Autodesk Inventor part; units mm, degrees
ref_plane "YZ Plane" through (0, 0, 0) normal (1, 0, 0) x (0, 1, 0)
ref_plane "XZ Plane" through (0, 0, 0) normal (0, 1, 0) x (-1, 0, 0)
ref_plane "XY Plane" through (0, 0, 0) normal (0, 0, 1) x (1, 0, 0)
sketch "스케치1" plane through (0, 0, 0) normal (0, 0, 1) x (1, 0, 0)
  line L0 (0, 0) -> (-35.14, 0)
  line L1 (-35.14, 0) -> (61.6, 0)
  line L2 (0, 35.14) -> (0, -35.14)
  line L3 (-35.14, -35.14) -> (61.6, -35.14)
  line L4 (61.6, -35.14) -> (61.6, 35.14)
  line L5 (61.6, 35.14) -> (-35.14, 35.14)
  line L6 (-35.14, 35.14) -> (-35.14, -35.14)
  line L7 (0, 0) -> (-27.87, 0)
  line L8 (0, 0) -> (42, 0)
  line L9 (42, 20) -> (42, -20)
  circle A0 centre (42, -20) radius 1.25
  circle A1 centre (42, 20) radius 1.25
  line L10 (0, 0) -> (45.5, 0)
  circle A2 centre (45.5, 0) radius 9
  circle A3 centre (45.5, 0) radius 16.1
  circle A4 centre (42, -20) radius 3
  circle A5 centre (42, 20) radius 3
  line L11 (45.5, 0) -> (61.6, 0) construction
  line L12 (42, 20) -> (45, 20) construction
  line L13 (44.1213, 22.1213) -> (55.8489, 12.3333)
  line L14 (42, 23) -> (0, 35.14)
  line L15 (-27.87, 28) -> (-27.87, -28)
  circle A6 centre (-27.87, 28) radius 1.25
  circle A7 centre (-27.87, 28) radius 3
  circle A8 centre (-27.87, -28) radius 1.25
  circle A9 centre (-27.87, -28) radius 3
  line L16 (-27.87, 31) -> (0, 35.14)
  line L17 (-30.87, 28) -> (-35.14, 0)
  line L18 (44.1213, -22.1213) -> (55.8489, -12.3333)
  line L19 (42, -23) -> (0, -35.14)
  line L20 (-27.87, -31) -> (0, -35.14)
  line L21 (-30.87, -28) -> (-35.14, 0)
  dimension "d20" = 6
  dimension "d0" = 35.14
  dimension "d1" = 96.74
  dimension "d3" = 70.28
  dimension "d4" = 27.87
  dimension "d9" = 42
  dimension "d11" = 40
  dimension "d12" = 2.5
  dimension "d13" = 2.5
  dimension "d14" = 45.5
  dimension "d15" = 18
  dimension "d16" = 32.2
  dimension "d19" = 6
  dimension "d27" = 56
  dimension "d28" = 2.5
  dimension "d29" = 6
  dimension "d30" = 2.5
  dimension "d31" = 6
extrude "돌출1" add sketch "스케치1" along normal blind 5.5 contours L2 L20 A9 L15 L0 | L2 L14 A5 L9 A3 L1 | L0 L15 A7 L16 L2 | L1 A3 L9 A4 L19 L2 | L15 A9 L21 L0 | L0 L17 A7 L15 | A3 L9 A2 L1 | L1 A2 L9 A3 | A3 L1 A2 L9 | L18 A4 L9 A3 | A7 | A9 | A2 L9 L1 | L1 L9 A2 | L9 A5 L13 A3 | L9 A2 L1 A3 | A5 | A4 | L9 A2 L1 | L1 A2 L9
sketch "스케치2" plane through (0, 0, 5.5) normal (0, 0, 1) x (1, 0, 0)
  line L0 (0, 0) -> (-35.14, 0)
  line L1 (-35.14, 0) -> (61.6, 0)
  line L2 (0, 35.14) -> (0, -35.14)
  line L3 (-35.14, -35.14) -> (61.6, -35.14)
  line L4 (61.6, -35.14) -> (61.6, 35.14)
  line L5 (61.6, 35.14) -> (-35.14, 35.14)
  line L6 (-35.14, 35.14) -> (-35.14, -35.14)
  line L7 (0, 0) -> (-27.87, 0)
  line L8 (0, 0) -> (42, 0)
  line L9 (42, 20) -> (42, -20)
  circle A0 centre (42, -20) radius 1.25
  circle A1 centre (42, 20) radius 1.25
  line L10 (0, 0) -> (45.5, 0)
  circle A2 centre (45.5, 0) radius 9
  circle A3 centre (45.5, 0) radius 16.1
  circle A4 centre (42, -20) radius 3
  circle A5 centre (42, 20) radius 3
  line L11 (45.5, 0) -> (61.6, 0) construction
  line L12 (42, 20) -> (45, 20) construction
  line L13 (44.1213, 22.1213) -> (55.8489, 12.3333)
  line L14 (42, 23) -> (0, 35.14)
  line L15 (-27.87, 28) -> (-27.87, -28)
  circle A6 centre (-27.87, 28) radius 1.25
  circle A7 centre (-27.87, 28) radius 3
  circle A8 centre (-27.87, -28) radius 1.25
  circle A9 centre (-27.87, -28) radius 3
  line L16 (-27.87, 31) -> (0, 35.14)
  line L17 (-30.87, 28) -> (-35.14, 0)
  line L18 (-27.87, -31) -> (0, -35.14)
  line L19 (-30.87, -28) -> (-35.14, 0)
  line L20 (42, -23) -> (0, -35.14)
  line L21 (44.1213, -22.1213) -> (55.8489, -12.3333)
  point P0 (55.7837, -12.3877)
  point P1 (55.7837, 12.3877)
  dimension "d46" = 6
  dimension "d34" = 35.14
  dimension "d35" = 96.74
  dimension "d36" = 70.28
  dimension "d37" = 27.87
  dimension "d38" = 42
  dimension "d39" = 40
  dimension "d40" = 2.5
  dimension "d41" = 2.5
  dimension "d42" = 45.5
  dimension "d43" = 18
  dimension "d44" = 32.2
  dimension "d45" = 6
  dimension "d47" = 56
  dimension "d48" = 2.5
  dimension "d49" = 6
  dimension "d50" = 2.5
  dimension "d51" = 6
extrude "돌출2" add sketch "스케치2" along normal blind 15 contours A3 L9 A2 L1 | L1 A2 L9 A3 | A3 L1 A2 L9 | A7 | A9 | A2 L9 L1 | L1 L9 A2 | L9 A2 L1 A3 | A5 | A4 | L9 A2 L1 | L1 A2 L9
sketch "스케치3" plane through (0, 0, 20.5) normal (0, 0, 1) x (1, 0, 0)
  line L0 (0, 0) -> (-35.14, 0)
  line L1 (-35.14, 0) -> (61.6, 0)
  line L2 (0, 35.14) -> (0, -35.14)
  line L3 (-35.14, -35.14) -> (61.6, -35.14)
  line L4 (61.6, -35.14) -> (61.6, 35.14)
  line L5 (61.6, 35.14) -> (-35.14, 35.14)
  line L6 (-35.14, 35.14) -> (-35.14, -35.14)
  line L7 (0, 0) -> (-27.87, 0)
  line L8 (0, 0) -> (42, 0)
  line L9 (42, 20) -> (42, -20)
  circle A0 centre (42, -20) radius 1.25
  circle A1 centre (42, 20) radius 1.25
  line L10 (0, 0) -> (45.5, 0)
  circle A2 centre (45.5, 0) radius 9
  circle A3 centre (45.5, 0) radius 16.1
  circle A4 centre (42, -20) radius 3
  circle A5 centre (42, 20) radius 3
  line L11 (45.5, 0) -> (61.6, 0) construction
  line L12 (42, 20) -> (45, 20) construction
  line L13 (44.1213, 22.1213) -> (55.8489, 12.3333)
  line L14 (42, 23) -> (0, 35.14)
  line L15 (-27.87, 28) -> (-27.87, -28)
  circle A6 centre (-27.87, 28) radius 1.25
  circle A7 centre (-27.87, 28) radius 3
  circle A8 centre (-27.87, -28) radius 1.25
  circle A9 centre (-27.87, -28) radius 3
  line L16 (-27.87, 31) -> (0, 35.14)
  line L17 (-30.87, 28) -> (-35.14, 0)
  line L18 (-27.87, -31) -> (0, -35.14)
  line L19 (-30.87, -28) -> (-35.14, 0)
  line L20 (42, -23) -> (0, -35.14)
  line L21 (44.1213, -22.1213) -> (55.8489, -12.3333)
  point P0 (42, -15.715)
  point P1 (55.7837, -12.3877)
  point P2 (55.7837, 12.3877)
  point P3 (42, 15.715)
  point P4 (42, 17)
  point P5 (42, -17)
  dimension "d66" = 6
  dimension "d54" = 35.14
  dimension "d55" = 96.74
  dimension "d56" = 70.28
  dimension "d57" = 27.87
  dimension "d58" = 42
  dimension "d59" = 40
  dimension "d60" = 2.5
  dimension "d61" = 2.5
  dimension "d62" = 45.5
  dimension "d63" = 18
  dimension "d64" = 32.2
  dimension "d65" = 6
  dimension "d67" = 56
  dimension "d68" = 2.5
  dimension "d69" = 6
  dimension "d70" = 2.5
  dimension "d71" = 6
extrude "돌출3" add sketch "스케치3" along normal blind 1.6 contours L2 L18 A9 L15 L0 | L2 L14 A5 L9 A3 L1 | L0 L15 A7 L16 L2 | L1 A3 L9 A4 L20 L2 | L15 A9 L19 L0 | L0 L17 A7 L15 | A3 L9 A2 L1 | L1 A2 L9 A3 | A3 L1 A2 L9 | A7 | A9 | A2 L9 L1 | L1 L9 A2 | L9 A2 L1 A3 | A5 | A4 | L9 A2 L1 | L1 A2 L9
sketch "스케치4" plane through (0, 0, 22.1) normal (0, 0, 1) x (1, 0, 0)
  line L0 (0, 0) -> (-35.14, 0)
  line L1 (-35.14, 0) -> (61.6, 0)
  line L2 (0, 35.14) -> (0, -35.14)
  line L3 (-35.14, -35.14) -> (61.6, -35.14)
  line L4 (61.6, -35.14) -> (61.6, 35.14)
  line L5 (61.6, 35.14) -> (-35.14, 35.14)
  line L6 (-35.14, 35.14) -> (-35.14, -35.14)
  line L7 (0, 0) -> (-27.87, 0)
  line L8 (0, 0) -> (42, 0)
  line L9 (42, 20) -> (42, -20)
  circle A0 centre (42, -20) radius 1.25
  circle A1 centre (42, 20) radius 1.25
  line L10 (0, 0) -> (45.5, 0)
  circle A2 centre (45.5, 0) radius 9
  circle A3 centre (45.5, 0) radius 16.1
  circle A4 centre (42, -20) radius 3
  circle A5 centre (42, 20) radius 3
  line L11 (45.5, 0) -> (61.6, 0) construction
  line L12 (42, 20) -> (45, 20) construction
  line L13 (44.1213, 22.1213) -> (55.8489, 12.3333)
  line L14 (42, 23) -> (0, 35.14)
  line L15 (-27.87, 28) -> (-27.87, -28)
  circle A6 centre (-27.87, 28) radius 1.25
  circle A7 centre (-27.87, 28) radius 3
  circle A8 centre (-27.87, -28) radius 1.25
  circle A9 centre (-27.87, -28) radius 3
  line L16 (-27.87, 31) -> (0, 35.14)
  line L17 (-30.87, 28) -> (-35.14, 0)
  line L18 (-27.87, -31) -> (0, -35.14)
  line L19 (-30.87, -28) -> (-35.14, 0)
  line L20 (42, -23) -> (0, -35.14)
  line L21 (44.1213, -22.1213) -> (55.8489, -12.3333)
  dimension "d86" = 6
  dimension "d74" = 35.14
  dimension "d75" = 96.74
  dimension "d76" = 70.28
  dimension "d77" = 27.87
  dimension "d78" = 42
  dimension "d79" = 40
  dimension "d80" = 2.5
  dimension "d81" = 2.5
  dimension "d82" = 45.5
  dimension "d83" = 18
  dimension "d84" = 32.2
  dimension "d85" = 6
  dimension "d87" = 56
  dimension "d88" = 2.5
  dimension "d89" = 6
  dimension "d90" = 2.5
  dimension "d91" = 6
extrude "돌출4" add sketch "스케치4" along normal blind 10 contours A7 | A9 | A5 | A4
sketch "스케치5" plane through (0, 0, 0) normal (0, 0, -1) x (-1, 0, 0)
  line L0 (27.87, -31) -> (0, -35.14)
  arc A0 (27.87, -31) -> (30.87, -28) centre (27.87, -28) ccw
  line L1 (35.14, 0) -> (30.87, -28)
  line L2 (30.87, 28) -> (35.14, 0)
  arc A1 (30.87, 28) -> (27.87, 31) centre (27.87, 28) ccw
  line L3 (0, 35.14) -> (27.87, 31)
  line L4 (-42, 23) -> (0, 35.14)
  arc A2 (-42, 23) -> (-44.1213, 22.1213) centre (-42, 20) ccw
  line L5 (-55.8489, 12.3333) -> (-44.1213, 22.1213)
  arc A3 (-55.8489, 12.3333) -> (-55.8489, -12.3333) centre (-45.5, 0) ccw
  line L6 (-44.1213, -22.1213) -> (-55.8489, -12.3333)
  arc A4 (-44.1213, -22.1213) -> (-42, -23) centre (-42, -20) ccw
  line L7 (0, -35.14) -> (-42, -23)
  circle A5 centre (-42, 20) radius 1.25
  circle A6 centre (27.87, 28) radius 1.25
  circle A7 centre (27.87, -28) radius 1.25
  circle A8 centre (-42, -20) radius 1.25
  line L8 (0, -35.14) -> (0, 35.14)
  line L9 (0, 0) -> (-45.5, 0)
  circle A9 centre (0, 0) radius 2.5
  circle A10 centre (-45.5, 0) radius 2.5
  dimension "d94" = 5
  dimension "d95" = 5
extrude "돌출5" add sketch "스케치5" along normal blind 2 contours A10 | A9 L9 L8 | L8 A9 | L9 A9 L8
sketch "스케치6" plane through (0, 0, 22.1) normal (0, 0, 1) x (1, 0, 0)
  arc A0 (42, -17) -> (42, -23) centre (42, -20) ccw
  line L0 (42, -17) -> (42, -15.715)
  arc A1 (42, -15.715) -> (55.7837, -12.3877) centre (45.5, 0) ccw
  line L1 (55.7837, -12.3877) -> (55.8489, -12.3333)
  arc A2 (55.8489, -12.3333) -> (55.8489, 12.3333) centre (45.5, 0) ccw
  line L2 (55.8489, 12.3333) -> (55.7837, 12.3877)
  arc A3 (55.7837, 12.3877) -> (42, 15.715) centre (45.5, 0) ccw
  line L3 (42, 15.715) -> (42, 17)
  arc A4 (42, 23) -> (42, 17) centre (42, 20) ccw
  line L4 (42, 23) -> (0, 35.14)
  line L5 (0, 35.14) -> (-27.87, 31)
  arc A5 (-30.87, 28) -> (-27.87, 31) centre (-27.87, 28) ccw
  line L6 (-30.87, 28) -> (-35.14, 0)
  line L7 (-35.14, 0) -> (-30.87, -28)
  arc A6 (-27.87, -31) -> (-30.87, -28) centre (-27.87, -28) ccw
  line L8 (-27.87, -31) -> (0, -35.14)
  line L9 (0, -35.14) -> (42, -23)
  circle A7 centre (-27.87, 28) radius 3
  circle A8 centre (-27.87, 28) radius 1.25
  circle A9 centre (-27.87, -28) radius 3
  circle A10 centre (-27.87, -28) radius 1.25
  circle A11 centre (42, -20) radius 1.25
  circle A12 centre (42, -20) radius 3
  circle A13 centre (42, -20) radius 1.25
  circle A14 centre (42, 20) radius 3
  circle A15 centre (42, 20) radius 1.25
  line L10 (-27.87, 28) -> (-27.87, 24.6)
  line L11 (-27.87, 24.6) -> (-9.87, 24.6)
  line L12 (-9.87, 24.6) -> (10.13, 24.6)
  line L13 (10.13, 24.6) -> (10.13, 29.6)
  line L14 (10.13, 29.6) -> (-9.87, 29.6)
  line L15 (-9.87, 29.6) -> (-9.87, 24.6)
  line L16 (-9.87, 29.6) -> (-7.87, 29.6)
  line L17 (-7.87, 29.6) -> (-9.87, 27.6)
  line L18 (10.13, 29.6) -> (8.13, 29.6)
  line L19 (8.13, 29.6) -> (10.13, 27.6)
  point P0 (0, 0)
  dimension "d98" = 3.4
  dimension "d99" = 18
  dimension "d100" = 20
  dimension "d101" = 5
  dimension "d102" = 2
  dimension "d103" = 45
  dimension "d104" = 2
extrude "돌출6" add sketch "스케치6" along normal blind 5 contours L15 L17 L14 L19 L13 L12
sketch "스케치7" plane through (0, 0, 27.1) normal (0, 0, 1) x (1, 0, 0)
  line L0 (8.13, 29.6) -> (-7.87, 29.6)
  line L1 (-7.87, 29.6) -> (-9.87, 27.6)
  line L2 (-9.87, 27.6) -> (-9.87, 24.6)
  line L3 (-9.87, 24.6) -> (10.13, 24.6)
  line L4 (10.13, 24.6) -> (10.13, 27.6)
  line L5 (10.13, 27.6) -> (8.13, 29.6)
  line L6 (-9.37, 27.3929) -> (-7.6629, 29.1)
  line L7 (-7.6629, 29.1) -> (7.9229, 29.1)
  line L8 (7.9229, 29.1) -> (9.63, 27.3929)
  line L9 (9.63, 27.3929) -> (9.63, 25.1)
  line L10 (9.63, 25.1) -> (-9.37, 25.1)
  line L11 (-9.37, 25.1) -> (-9.37, 27.3929)
  point P0 (0, 0)
  dimension "d107" = 0.5
extrude "돌출7" cut sketch "스케치7" against normal blind 5 contours L6 L7 L8 L9 L10 L11
properties part number "base"
Geometry check sheet. Reference: the model listing, model coordinates, mm. A direction names the side the tool comes from. Give positions to 0.01 mm unless a question says otherwise; leave off trailing zeros. Write each loop counter-clockwise with the first axis right and the second up, starting at its lowest first coordinate (ties: lowest second). Pieces come first, ordered by that corner, then holes. Notation, with made-up numbers: (51, -20.5) - (106, -20.5) arc R25 cw to (106, 1.5) - close; hole circle Ø6 at (-39.75, 20.5). An arc over 180 degrees is marked (long way). Put each result on its own line as item: value.
1. Draft check along X on faces 1 (the flat face through (-8.86, 28.61, 24.56)), 2 (the flat face through (46, 0, -2)), 3 (the flat face through (-14.13, -33.04, 2.71)), 4 (the flat face through (10.13, 26, 25)). Enter one of: +X half, -X half, draft (parallel to the pull), parting line (faces both ways), or undercut.
Ans:
face 1: undercut
face 2: draft
face 3: -X half
face 4: +X half
2. Sectioned sample at A-A, the plane z = 10. Give the number of separate pieces and of enclosed holes in the cut face, plus the area to 3 significant figures.
Ans:
separate pieces: 5
enclosed holes: 4
area: 908 mm²
3. Sectioned sample at B-B, the plane x = -15. Enter the section's corners in (y, z), plus the area to 3 significant figures.
Ans:
outline: (-32.91, 0) - (32.91, 0) - (32.91, 5.5) - (-32.91, 5.5) - close; (-32.91, 20.5) - (32.91, 20.5) - (32.91, 22.1) - (-32.91, 22.1) - close
area: 467 mm²
4. Sectioned sample at D-D, the plane z = 4. Enter the section's corners in (x, y), plus the area to 3 significant figures.
Ans:
outline: (-35.14, 0) - (-30.87, -28) arc R3 ccw to (-27.87, -31) - (0, -35.14) - (42, -23) arc R3 ccw to (44.12, -22.12) - (55.85, -12.33) arc R16.1 ccw to (55.85, 12.33) - (44.12, 22.12) arc R3 ccw to (42, 23) - (0, 35.14) - (-27.87, 31) arc R3 ccw to (-30.87, 28) - close; hole circle Ø2.5 at (-27.87, -28); hole circle Ø2.5 at (-27.87, 28); hole circle Ø2.5 at (42, -20); hole circle Ø2.5 at (42, 20)
area: 5,170 mm²
5. Set-up check for faces 5 (the flat face through (0, 29.6, 25)), 6 (the flat face through (9.63, 26, 25)), 7 (the cylindrical face through (-30.08, -30.03, 19.39)), 8 (the flat face through (21.294, -28.985, 21.289)): record each of +Z, -Z, +X, -X, +Y, -Y from which the full face is reachable in a straight line by a thin tool's end or side.
Ans:
face 5: +Z, +X, +Y
face 6: +Z
face 7: none
face 8: +Z, -Z, +X, -Y
6. Thickness scan on line 1 (Y direction, x = -27.87, z = 18); line 2 (Y direction, x = 42, z = 18.5); line 3 (X direction, y = -20, z = 17.5). Record the ranges inside material, lowest first.
Ans:
line 1: y = -31 to -29.25, -26.75 to -25, 25 to 26.75, 29.25 to 31
line 2: y = -23 to -21.25, -18.75 to -17, -15.71 to 15.71, 17 to 18.75, 21.25 to 23
line 3: x = 39 to 40.75, 43.25 to 45
7. Go/stop test with flat-tipped pins: pin 1 (1.1 mm diameter, centred on y = 26.5, z = 24.5, fed in from -X); pin 2 (1.5 mm diameter, centred on y = 26.5, z = 25.5, fed in from +X); pin 3 (6 mm diameter, centred on y = -17.5, z = 11.5, fed in from +X). Record where each tip stops, or that it passes through.
Ans:
pin 1: stops at x = -30.72
pin 2: stops at x = 10.13
pin 3: stops at x = 52.5
8. Sectioned sample at C-C, the plane y = -7.5. Enter the section's corners in (x, z).
Ans:
outline: (-34, 0) - (59.75, 0) - (59.75, 22.1) - (-34, 22.1) - (-34, 20.5) - (31.25, 20.5) - (31.25, 5.5) - (-34, 5.5) - close
